Here's how the part is built. I have some questions about the finished solid (model axes, mm). Round coordinates to 2 decimals unless told otherwise and drop trailing zeros. Order: outer loops, then holes, each group sorted by start corner. A loop starts at its lowest first (then second) coordinate and runs counter-clockwise, first axis right, second up. Notation, with made-up numbers: (65, 14.5) -> (116, 14.5) arc R10 ccw to (116, 19.5) -> close; hole circle Ø10 at (33.5, 12.5). An arc over 180 degrees is marked (long way). One line per item, written item: value.
```python
from build123d import *

# Parameters (mm, degrees)
SKETCH_1_W          = 290
SKETCH_1_H          = 45
EXTRUDE_1_DEPTH     = 2
SKETCH_3_R          = 2.025
CUT_EXTRUDE_1_DEPTH = 10
SKETCH_4_R          = 2
CUT_EXTRUDE_2_DEPTH = 10
SKETCH_5_R          = 2
CUT_EXTRUDE_3_DEPTH = 35
SKETCH_6_W          = 47.500000831
SKETCH_6_H          = 33
CUT_EXTRUDE_4_DEPTH = 129.5
SKETCH_7_W          = 84.999998338
SKETCH_7_H          = 33
CUT_EXTRUDE_5_DEPTH = 129.5
FILLET_1_R          = 2
FILLET_2_R          = 2


with BuildPart() as part:
    # 草图1 → 凸台-拉伸1 (new, symmetric)
    with BuildSketch(Plane.XY):
        Rectangle(SKETCH_1_W, SKETCH_1_H)
    extrude(amount=EXTRUDE_1_DEPTH, both=True)

    # 草图3 → 切除-拉伸1 (cut)
    with BuildSketch(Plane(origin=(0, 0, -2), x_dir=(-1, 0, 0), z_dir=(0, 0, -1))):
        with Locations((-47.499999169, 8.524320115)):
            Circle(SKETCH_3_R)
        with Locations((-47.499999169, -16.475679885)):
            Circle(SKETCH_3_R)
        with Locations((47.500000831, 8.524320115)):
            Circle(SKETCH_3_R)
        with Locations((47.500000831, -16.475679885)):
            Circle(SKETCH_3_R)
    extrude(amount=-CUT_EXTRUDE_1_DEPTH, mode=Mode.SUBTRACT)

    # 草图4 → 切除-拉伸2 (cut)
    with BuildSketch(Plane(origin=(0, 0, -2), x_dir=(-1, 0, 0), z_dir=(0, 0, -1))):
        with Locations((-130, 15)):
            Circle(SKETCH_4_R)
        with Locations((-130, -15)):
            Circle(SKETCH_4_R)
    cut_extrude_2 = extrude(amount=-CUT_EXTRUDE_2_DEPTH, mode=Mode.SUBTRACT)

    # 镜向1: 切除-拉伸2 across plane
    add(cut_extrude_2.mirror(Plane(origin=(0, 0, 0), x_dir=(0, 0, 1), z_dir=(1, 0, 0))), mode=Mode.SUBTRACT)

    # 草图5 → 切除-拉伸3 (cut, symmetric)
    with BuildSketch(Plane(origin=(0, 0, -2), x_dir=(-1, 0, 0), z_dir=(0, 0, -1))):
        with Locations((-105, -17.5)):
            Circle(SKETCH_5_R)
        with Locations((-105, 12.5)):
            Circle(SKETCH_5_R)
    cut_extrude_3 = extrude(amount=CUT_EXTRUDE_3_DEPTH, both=True, mode=Mode.SUBTRACT)

    # 镜向2: 切除-拉伸3 across plane
    add(cut_extrude_3.mirror(Plane(origin=(0, 0, 0), x_dir=(0, 0, 1), z_dir=(1, 0, 0))), mode=Mode.SUBTRACT)

    # 草图6 → 切除-拉伸4 (cut, symmetric)
    with BuildSketch(Plane(origin=(0, 0, -2), x_dir=(-1, 0, 0), z_dir=(0, 0, -1))):
        with Locations((-76.249999585, 0)):
            Rectangle(SKETCH_6_W, SKETCH_6_H)
    cut_extrude_4 = extrude(amount=CUT_EXTRUDE_4_DEPTH, both=True, mode=Mode.SUBTRACT)

    # 镜向3: 切除-拉伸4 across plane
    add(cut_extrude_4.mirror(Plane(origin=(0, 0, 0), x_dir=(0, 0, 1), z_dir=(1, 0, 0))), mode=Mode.SUBTRACT)

    # 草图7 → 切除-拉伸5 (cut, symmetric)
    with BuildSketch(Plane(origin=(0, 0, -2), x_dir=(-1, 0, 0), z_dir=(0, 0, -1))):
        Rectangle(SKETCH_7_W, SKETCH_7_H)
    extrude(amount=CUT_EXTRUDE_5_DEPTH, both=True, mode=Mode.SUBTRACT)

    # 圆角1
    fillet_1_edges = [part.edges().sort_by_distance(p)[0] for p in [
        (-52.499999169, -16.5, 0),
        (-52.499999169, 16.5, 0),
        (-100, 16.5, 0),
        (-100, -16.5, 0),
        (-42.499999169, 16.5, 0),
        (-42.499999169, -16.5, 0),
        (42.499999169, -16.5, 0),
        (42.499999169, 16.5, 0),
        (52.499999169, 16.5, 0),
        (52.499999169, -16.5, 0),
        (100, -16.5, 0),
        (100, 16.5, 0),
    ]]
    fillet(fillet_1_edges, radius=FILLET_1_R)

    # 圆角2
    fillet_2_edges = [part.edges().sort_by_distance(p)[0] for p in [
        (145, -22.5, 0),
        (-145, -22.5, 0),
        (-145, 22.5, 0),
        (145, 22.5, 0),
    ]]
    fillet(fillet_2_edges, radius=FILLET_2_R)


solid = part.part
```
Q1. I want a section at B-B on x = 20.5. Write out the boundary of the cut face in (y, z), then the cut area to 3 significant figures.
Answers:
outline: (-22.5, -2) -> (-16.5, -2) -> (-16.5, 2) -> (-22.5, 2) -> close; (16.5, -2) -> (22.5, -2) -> (22.5, 2) -> (16.5, 2) -> close
area: 48.0 mm2
Q2. I want a section at C-C on z = 0.2. Give the number of separate pieces and of enclosed holes in the cut face, then the cut area to 3 significant figures.
Answers:
separate pieces: 1
enclosed holes: 15
area: 6,960 mm2
Q3. If we mould it in two halves opening along Z, with no side actions, what happens to faces 1 (the face through (-2, -20, -2)), 2 (the face through (-2, -20, 2))? For each: pulls with the +Z half, pulls with the -Z half, needs draft (parallel to the pull), parting line crosses it, or undercut.
Answers:
face 1: pulls with the -Z half
face 2: pulls with the +Z half
Q4. I want a section at A-A on y = -5.5. Write out the boundary of the cut face in (x, z), then the cut area to 3 significant figures.
Answers:
outline: (-145, -2) -> (-100, -2) -> (-100, 2) -> (-145, 2) -> close; (-52.5, -2) -> (-42.5, -2) -> (-42.5, 2) -> (-52.5, 2) -> close; (42.5, -2) -> (52.5, -2) -> (52.5, 2) -> (42.5, 2) -> close; (100, -2) -> (145, -2) -> (145, 2) -> (100, 2) -> close
area: 440 mm2
Q5. I need wall thicknesses on line 1 along Y through (x, z) = (105, 0.9); line 2 along X through (y, z) = (1, -0.05); line 3 along Y through (x, z) = (-130, 0.85). Which ranges of each line are inside material? Lowest first, please.
Answers:
line 1: -22.5 to -19.5, -15.5 to 10.5, 14.5 to 22.5
line 2: -145 to -100, -52.5 to -42.5, 42.5 to 52.5, 100 to 145
line 3: -22.5 to -17, -13 to 13, 17 to 22.5
